```python
from build123d import *

# Parameters (mm, degrees)
BOSS_EXTRUDE1_DEPTH      = 11
BOSS_EXTRUDE1_DEPTH_BACK = 11
CUT_EXTRUDE1_DEPTH       = 0.5
CUT_EXTRUDE2_DEPTH       = 5
CUT_EXTRUDE3_DEPTH       = 5
CUT_EXTRUDE4_DEPTH       = 0.5
CUT_EXTRUDE5_DEPTH       = 0.5
CUT_EXTRUDE6_DEPTH       = 0.5
CUT_EXTRUDE7_DEPTH       = 0.5
CUT_EXTRUDE8_DEPTH       = 1
CUT_EXTRUDE8_DEPTH_BACK  = 1


with BuildPart() as part:
    # Sketch1 → Boss-Extrude1 (new body, two sides)
    with BuildSketch(Plane.XY) as boss_extrude1_sk:
        with BuildLine():
            Line((0, 9.8), (0, -14.1))
            Line((0, -14.1), (0.5, -14.1))
            Line((0.5, -14.1), (0.5, 9.8))
            ThreePointArc((0.5, 9.8), (2.126963265, 11.294617118), (3.478507106, 9.546984708))
            Line((3.478507106, 9.546984708), (0.580460074, -7.387893417))
            ThreePointArc((0.580460074, -7.387893417), (0.597810426, -7.717762239), (0.75519649, -8.008182798))
            Line((0.75519649, -8.008182798), (4.700431296, -12.518581837))
            Line((4.700431296, -12.518581837), (5.076776054, -12.189394014))
            Line((5.076776054, -12.189394014), (1.131541248, -7.678994975))
            ThreePointArc((1.131541248, -7.678994975), (1.079079227, -7.582188122), (1.073295776, -7.472231848))
            Line((1.073295776, -7.472231848), (3.971342808, 9.462646278))
            ThreePointArc((3.971342808, 9.462646278), (2.169284353, 11.792822824), (0, 9.8))
        make_face()
    extrude(amount=BOSS_EXTRUDE1_DEPTH)
    extrude(boss_extrude1_sk.sketch, amount=-BOSS_EXTRUDE1_DEPTH_BACK)

    # Sketch2 → Cut-Extrude1 (cut)
    with BuildSketch(Plane(origin=(0, 0, 0), x_dir=(0, 0, -1), z_dir=(1, 0, 0))):
        with BuildLine():
            Line((-4.5, 0), (-4.5, -14.1))
            Line((-4.5, -14.1), (4.5, -14.1))
            Line((4.5, -14.1), (4.5, 0))
            ThreePointArc((4.5, 0), (0, 4.5), (-4.5, 0))
        make_face()
    extrude(amount=CUT_EXTRUDE1_DEPTH, mode=Mode.SUBTRACT)

    # Sketch3 → Cut-Extrude2 (cut)
    with BuildSketch(Plane(origin=(0.5, 0, 0), x_dir=(0, 0, -1), z_dir=(1, 0, 0))):
        with BuildLine():
            Line((5.948789681, 0.782241223), (4.5, 11.8))
            Line((4.5, 11.8), (-4.5, 11.8))
            Line((-4.5, 11.8), (-5.948789681, 0.782241223))
            ThreePointArc((-5.948789681, 0.782241223), (0, -6), (5.948789681, 0.782241223))
        make_face()
    extrude(amount=CUT_EXTRUDE2_DEPTH, mode=Mode.SUBTRACT)

    # Sketch4 → Cut-Extrude3 (cut)
    with BuildSketch(Plane(origin=(0.5, 0, 0), x_dir=(0, 0, -1), z_dir=(1, 0, 0))):
        with BuildLine():
            Line((4.834801398, 9.253901634), (4.5, 11.8))
            Line((4.5, 11.8), (-4.5, 11.8))
            Line((-4.5, 11.8), (-4.834801398, 9.253901634))
            ThreePointArc((-4.834801398, 9.253901634), (-4.449655576, 8.328306669), (-3.455120629, 8.20195961))
            ThreePointArc((-3.455120629, 8.20195961), (1.1e-08, 8.9), (3.455120648, 8.201959602))
            ThreePointArc((3.455120648, 8.201959602), (4.449655585, 8.328306676), (4.834801398, 9.253901634))
        make_face()
    extrude(amount=-CUT_EXTRUDE3_DEPTH, mode=Mode.SUBTRACT)

    # Sketch5 → Cut-Extrude4 (cut)
    with BuildSketch(Plane(origin=(0, 0, 0), x_dir=(0, 0, -1), z_dir=(1, 0, 0))):
        with BuildLine():
            Line((-11, -14.1), (-7, -14.1))
            ThreePointArc((-7, -14.1), (-9.828427125, -12.928427125), (-11, -10.1))
            Line((-11, -10.1), (-11, -14.1))
        make_face()
    extrude(amount=CUT_EXTRUDE4_DEPTH, mode=Mode.SUBTRACT)

    # Sketch6 → Cut-Extrude5 (cut)
    with BuildSketch(Plane(origin=(0, 0, 0), x_dir=(0, 0, -1), z_dir=(1, 0, 0))):
        with BuildLine():
            Line((7, -14.1), (11, -14.1))
            Line((11, -14.1), (11, -10.1))
            ThreePointArc((11, -10.1), (9.828427125, -12.928427125), (7, -14.1))
        make_face()
    extrude(amount=CUT_EXTRUDE5_DEPTH, mode=Mode.SUBTRACT)

    # Sketch7 → Cut-Extrude6 (cut)
    with BuildSketch(Plane(origin=(0, 0, 0), x_dir=(0, 0, -1), z_dir=(1, 0, 0))):
        with BuildLine():
            Line((4.5, -14.1), (5.5, -14.1))
            ThreePointArc((5.5, -14.1), (4.792893219, -13.807106781), (4.5, -13.1))
            Line((4.5, -13.1), (4.5, -14.1))
        make_face()
    extrude(amount=CUT_EXTRUDE6_DEPTH, mode=Mode.SUBTRACT)

    # Sketch8 → Cut-Extrude7 (cut)
    with BuildSketch(Plane(origin=(0, 0, 0), x_dir=(0, 0, -1), z_dir=(1, 0, 0))):
        with BuildLine():
            Line((-5.5, -14.1), (-4.5, -14.1))
            Line((-4.5, -14.1), (-4.5, -13.1))
            ThreePointArc((-4.5, -13.1), (-4.792893219, -13.807106781), (-5.5, -14.1))
        make_face()
    extrude(amount=CUT_EXTRUDE7_DEPTH, mode=Mode.SUBTRACT)

    # Sketch9 → Cut-Extrude8 (cut, two sides)
    with BuildSketch(Plane(origin=(-3.164279663, -2.76778754, 0), x_dir=(0, 0, -1), z_dir=(0.752689517, 0.658375646, 0))) as cut_extrude8_sk:
        with BuildLine():
            Line((-11, -8.516878218), (-15, -8.516878218))
            Line((-15, -8.516878218), (-15, -16.516878218))
            Line((-15, -16.516878218), (15, -16.516878218))
            Line((15, -16.516878218), (15, -8.516878218))
            Line((15, -8.516878218), (11, -8.516878218))
            ThreePointArc((11, -8.516878218), (9.828427125, -11.345305343), (7, -12.516878218))
            Line((7, -12.516878218), (-7, -12.516878218))
            ThreePointArc((-7, -12.516878218), (-9.828427125, -11.345305343), (-11, -8.516878218))
        make_face()
    extrude(amount=CUT_EXTRUDE8_DEPTH, mode=Mode.SUBTRACT)
    extrude(cut_extrude8_sk.sketch, amount=-CUT_EXTRUDE8_DEPTH_BACK, mode=Mode.SUBTRACT)


solid = part.part
```
Input: part model. Units: mm. Frame: model coordinates. A direction names the side the tool comes from. Coordinates: 2 decimals unless noted, no trailing zeros. Write each loop counter-clockwise with the first axis right and the second up, starting at its lowest first coordinate (ties: lowest second). Pieces come first, ordered by that corner, then holes. Notation, with made-up numbers: (-16.5, 35) -> (27.5, 35) arc R29 ccw to (27.5, 55) -> close; hole circle Ø11 at (38, 82). An arc over 180 degrees is marked (long way). Answer as a JSON object with one key per item and string values.
1. Section B-B on y = -11.5. Count the separate pieces of the cut face and the enclosed holes in it, then the cut area to 3 significant figures.
Result set:
{"separate pieces": "3", "enclosed holes": "0", "area": "19.2 mm2"}
2. Material intervals for line 1 (X direction, y = 9.8, z = 7); line 2 (X direction, y = -5, z = 7); line 3 (Z direction, x = 1.5, y = -4), sorted ascending. Write a range as from..to.
Result set:
{"line 1": "x = 0..0.5, 3.5..4", "line 2": "x = 0..0.5, 0.99..1.5", "line 3": "z = -11..-4.47, 4.47..11"}
3. Section C-C on z = 2.25. Return the cut outline in (x, y).
Result set:
{"outline": "(0, 3.9) -> (0.5, 3.9) -> (0.5, 8.61) -> (0, 8.61) -> close; (0.58, -7.39) arc R0.75 ccw to (0.76, -8.01) -> (4.7, -12.52) -> (5.08, -12.19) -> (1.13, -7.68) arc R0.25 cw to (1.07, -7.47) -> (1.4, -5.56) -> (0.89, -5.56) -> close"}
4. First-contact query: P1, Ø1.5, axis at x = 4, z = 1.5, coming from the +Y side; P2, Ø2.5, axis at x = 2, y = 9.8, coming from the -Z side; P3, Ø11, axis at y = 2, z = -4, coming from the +X side; P4, Ø2, axis at x = 4, y = -10.5, coming from the -Z side. Flat tips, straight axial feed; report the tip coordinate or a pass-through.
Result set:
{"P1": "stops at y = -10.1", "P2": "passes through", "P3": "stops at x = 3.62", "P4": "stops at z = -10.86"}
5. Section A-A on z = 0. Return the cut outline in (x, y), then the cut area to 3 significant figures.
Result set:
{"outline": "(0, 4.5) -> (0.5, 4.5) -> (0.5, 8.9) -> (0, 8.9) -> close; (0.58, -7.39) arc R0.75 ccw to (0.76, -8.01) -> (4.7, -12.52) -> (5.08, -12.19) -> (1.13, -7.68) arc R0.25 cw to (1.07, -7.47) -> (1.33, -6) -> (0.82, -6) -> close", "area": "6.14 mm2"}
6. Access query for faces 1 (the face through (1, -6, 0)), 2 (the face through (0.246, -13.799, 4.785)), 3 (the face through (0.5, -2, 5)). Directions: +Z, -Z, +X, -X, +Y, -Y. A direction counts if a zero-diameter tool reaches every point of the face in a straight line with its end or side. Return the directions, or none.
Result set:
{"face 1": "+X", "face 2": "+X, -X, -Y", "face 3": "+Z, -Z, -Y"}
7. Mould query, pull axis Z, two halves, no side actions, for faces 4 (the face through (0.2, 4.5, -0.1)), 5 (the face through (2.7, -10.23, 0.15)), 6 (the face through (2.4, 1.7, -11)). Classes: released by +Z, released by -Z, zero draft, split by the parting line, or undercut.
Result set:
{"face 4": "undercut", "face 5": "zero draft", "face 6": "released by -Z"}
